Autodesk Inventor part; units mm, degrees
ref_plane "YZ Plane" through (0, 0, 0) normal (1, 0, 0) x (0, 1, 0)
ref_plane "XZ Plane" through (0, 0, 0) normal (0, 1, 0) x (-1, 0, 0)
ref_plane "XY Plane" through (0, 0, 0) normal (0, 0, 1) x (1, 0, 0)
sketch "Sketch1" plane through (0, 0, 0) normal (1, 0, 0) x (0, 1, 0)
  line L0 (-2.71, -15.0951) -> (7.29, -15.0951)
  line L1 (7.29, -15.0951) -> (7.29, 34.9049)
  line L2 (7.29, 34.9049) -> (-2.71, 34.9049)
  line L3 (-2.71, 34.9049) -> (-2.71, -15.0951)
  point P0 (0, 0)
  dimension "d0" = 50
  dimension "d1" = 10
extrude "Extrusion1" add sketch "Sketch1" along normal blind 30
sketch "Sketch2" plane through (0, 0, 0) normal (1, 0, 0) x (0, 1, 0)
  line L0 (7.29, -15.0951) -> (7.29, 34.9049)
  line L1 (7.29, -15.0951) -> (32.29, -15.0951)
  line L2 (32.29, -15.0951) -> (32.29, 4.9049)
  line L3 (32.29, 4.9049) -> (7.29, 4.9049)
  point P0 (0, 0)
  dimension "d4" = 25
  dimension "d5" = 20
extrude "Extrusion2" add sketch "Sketch2" along normal blind 10
sketch "Sketch3" plane through (30, 0, 0) normal (1, 0, 0) x (0, 0, -1)
  line L0 (-34.9049, 7.29) -> (-34.9049, -2.71)
  line L1 (-34.9049, 7.29) -> (-34.9049, 17.29)
  line L2 (-34.9049, 17.29) -> (-14.9049, 17.29)
  line L3 (-14.9049, 17.29) -> (-14.9049, 7.29)
  line L4 (15.0951, 7.29) -> (-34.9049, 7.29)
  line L5 (-14.9049, 7.29) -> (-34.9049, 7.29)
  point P0 (0, 0)
  dimension "d8" = 20
  dimension "d9" = 10
extrude "Extrusion3" add sketch "Sketch3" against normal blind 10
properties part number "BT004_Formstück"
Work out the finished part from the listing and answer in its coordinate system (mm). A direction names the side the tool comes from. Give positions to 0.01 mm unless a question says otherwise; leave off trailing zeros. Order: outer loops, then holes, each group sorted by start corner. A loop starts at its lowest first (then second) coordinate and runs counter-clockwise, first axis right, second up.
1. Section D-D, the plane z = 8.5 is taken. Determine the outline of the cut face in (x, y).
Result sheet:
outline: (0, -2.71) - (30, -2.71) - (30, 7.29) - (0, 7.29) - close
2. For faces 1 (the flat face through (20, 12, 25)), 2 (the flat face through (25, 12, 14.905)), 3 (the flat face through (5, 20, 4.905)), 4 (the flat face through (10, 20, -5)), determine the directions among +Z, -Z, +X, -X, +Y, -Y from which every point of the face is accessible in a straight line to the end or side of a thin tool.
Result sheet:
face 1: +Z, -Z, -X, +Y
face 2: -Z, +X, -X, +Y
face 3: +Z, +X, -X, +Y
face 4: +Z, -Z, +X, +Y
3. Section A-A, the plane y = 11 is taken. Determine the outline of the cut face in (x, z), and give its area (3 significant figures).
Result sheet:
outline: (0, -15.1) - (10, -15.1) - (10, 4.9) - (0, 4.9) - close; (20, 14.9) - (30, 14.9) - (30, 34.9) - (20, 34.9) - close
area: 400 mm2
4. Each of these flat-tipped pins is pushed along its axis until it touches: P1, Ø1, axis at x = 4.5, y = 20, coming from the +Z side; P2, Ø1.5, axis at x = 11.5, y = 28.5, coming from the +Z side; P3, Ø5, axis at x = 9, z = 9, coming from the +Y side; P4, Ø3, axis at x = 25.5, y = 10.5, coming from the -Z side. Where does it stop, or does it pass through?
Result sheet:
P1: stops at z = 4.9
P2: passes through
P3: stops at y = 7.29
P4: stops at z = 14.9
5. Section B-B, the plane z = 30 is taken. Determine the outline of the cut face in (x, y), and give its area (3 significant figures).
Result sheet:
outline: (0, -2.71) - (30, -2.71) - (30, 17.29) - (20, 17.29) - (20, 7.29) - (0, 7.29) - close
area: 400 mm2
6. Straight lines are drawn through the part: L1, parallel to Z at x = 7.75, y = 10; L2, parallel to X at y = 9, z = 16; L3, parallel to X at y = 26.5, z = -1. For each, find the intervals that lie inside material, in ascending order.
Result sheet:
L1: z = -15.1 to 4.9
L2: x = 20 to 30
L3: x = 0 to 10
7. Section C-C, the plane x = 23.5 is taken. Determine the outline of the cut face in (y, z), and give its area (3 significant figures).
Result sheet:
outline: (-2.71, -15.1) - (7.29, -15.1) - (7.29, 14.9) - (17.29, 14.9) - (17.29, 34.9) - (-2.71, 34.9) - close
area: 700 mm2
